Could you check a few things on this model? Use its own coordinates, in mm. A direction names the side the tool comes from. Coordinates: 2 decimals unless noted, no trailing zeros. Loops run counter-clockwise (first coordinate to the right, second up) from the corner with the lowest first, then second, coordinate; pieces in that order, holes last.
from build123d import *

# Parameters (mm, degrees)
F2_R          = 4
F3_DEPTH      = 25
F3_DEPTH_BACK = 25


with BuildPart() as f1:
    # F0 (on Front) → F1 (revolve)
    with BuildSketch(Plane.XZ):
        Polygon((-8, 0), (0, 0), (0, 13), (-8, 13), (-16, 13), (-16, 11.2221399145), (-11.3175004572, 9), (-16, 6.7778600855), (-16, 5), (-8, 5), align=None)
    revolve(axis=Axis((0, 0, 6.5), (0, 0, -1)))

    # F2 (on Top) → F3 (cut, two sides)
    with BuildSketch(Plane.XY) as f3_sk:
        Circle(F2_R)
    extrude(amount=-F3_DEPTH, mode=Mode.SUBTRACT)
    extrude(f3_sk.sketch, amount=F3_DEPTH_BACK, mode=Mode.SUBTRACT)


solid = f1.part
(1) Which directions (+Z, -Z, +X, -X, +Y, -Y) give clear straight access to the entire face, cutting with the end or side of a thin tool? Please do faces 4 (the face through (3.8, 7.3, 5)), 5 (the face through (9.214, -7.065, 8.861)), 6 (the face through (3.47, -15.62, 12.1)).
Answers:
face 4: -Z
face 5: none
face 6: +Z, -Z
(2) Imagine slicing it at C-C, the plane z = 7.5. Write out the boundary of the cut face in (x, y).
Answers:
outline: circle Ø28.96 at (0, 0); hole circle Ø8 at (0, 0)
(3) We'd pull the mould along X, two halves only. Please class faces 1 (the face through (-0.867, -3.905, 6.409)), 2 (the face through (4, -2, 0)), 3 (the face through (1.73, -7.81, 2.46)): +X half, -X half, draft (parallel to the pull), parting line (faces both ways), or undercut.
Answers:
face 1: undercut
face 2: draft
face 3: parting line
(4) Imagine slicing it at A-A, the plane x = 0. Write out the boundary of the cut face in (y, z), and give its area (3 significant figures).
Answers:
outline: (-16, 5) - (-8, 5) - (-8, 0) - (-4, 0) - (-4, 13) - (-16, 13) - (-16, 11.22) - (-11.32, 9) - (-16, 6.78) - close; (4, 0) - (8, 0) - (8, 5) - (16, 5) - (16, 6.78) - (11.32, 9) - (16, 11.22) - (16, 13) - (4, 13) - close
area: 211 mm2
(5) For pin 1 (5 mm diameter, centred on x = -12, y = 3.5, fed in from -Z); pin 2 (1 mm diameter, centred on x = -7.5, z = 3.5, fed in from +Y); pin 3 (12 mm diameter, centred on x = -8.5, y = -10.5, fed in from -Z); pin 4 (6 mm diameter, centred on y = -12, z = 6, fed in from -X), each with a flat end and sliding along its axis, tell me the tip position at first contact or that it passes through.
Answers:
pin 1: stops at z = 5
pin 2: stops at y = 3.87
pin 3: stops at z = 0
pin 4: stops at x = -13.23
(6) I need wall thicknesses on probe 1 along Y at (x, z) = (0, 3.5); probe 2 along Y at (x, z) = (0, 6.5); probe 3 along Z at (x, y) = (9, 4). Which ranges of each line are inside material? Lowest first, please.
Answers:
probe 1: y = -8 to -4, 4 to 8
probe 2: y = -16 to -4, 4 to 16
probe 3: z = 5 to 13
